Geometry: final body of the model. Coordinates: model frame, mm. A direction names the side the tool comes from. Give positions to 0.01 mm unless a question says otherwise; leave off trailing zeros. Write each loop counter-clockwise with the first axis right and the second up, starting at its lowest first coordinate (ties: lowest second). Pieces come first, ordered by that corner, then holes.
```python
from build123d import *

# Parameters (mm, degrees)
SKETCH1_W           = 96.52
SKETCH1_H           = 72.39
BOSS_EXTRUDE1_DEPTH = 5.08
SHELL1_T            = -2.667
FILLET1_R           = 6.35
FILLET2_R           = 8.89
SKETCH2_W           = 36.83
SKETCH2_H           = 2.413
CUT_EXTRUDE1_DEPTH  = 5.08
SKETCH3_W           = 17.78
SKETCH3_H           = 2.413
CUT_EXTRUDE2_DEPTH  = 5.08
FILLET3_R           = 0.508
CUT_EXTRUDE3_REACH  = 7.08
SKETCH4_R           = 3.25
CUT_EXTRUDE4_DEPTH  = 6.08


with BuildPart() as part:
    # Sketch1 → Boss-Extrude1 (new body)
    with BuildSketch(Plane(origin=(0, 0, 0), x_dir=(1, 0, 0), z_dir=(0, 1, 0))):
        Rectangle(SKETCH1_W, SKETCH1_H)
    extrude(amount=BOSS_EXTRUDE1_DEPTH)

    # Shell1
    shell1_openings = [part.faces().sort_by_distance(p)[0] for p in [
        (0, 5.08, 0),
    ]]
    offset(amount=SHELL1_T, openings=shell1_openings, kind=Kind.INTERSECTION)

    # Fillet1
    fillet1_edges = [part.edges().sort_by_distance(p)[0] for p in [
        (45.593, 3.8735, 33.528),
        (45.593, 3.8735, -33.528),
        (-45.593, 3.8735, -33.528),
        (-45.593, 3.8735, 33.528),
    ]]
    fillet(fillet1_edges, radius=FILLET1_R)

    # Fillet2
    fillet2_edges = [part.edges().sort_by_distance(p)[0] for p in [
        (48.26, 2.54, 36.195),
        (-48.26, 2.54, 36.195),
        (-48.26, 2.54, -36.195),
        (48.26, 2.54, -36.195),
    ]]
    fillet(fillet2_edges, radius=FILLET2_R)

    # Sketch2 → Cut-Extrude1 (cut)
    with BuildSketch(Plane.XY.offset(36.195)):
        with Locations((17.145, 3.8735)):
            Rectangle(SKETCH2_W, SKETCH2_H)
    extrude(amount=-CUT_EXTRUDE1_DEPTH, mode=Mode.SUBTRACT)

    # Sketch3 → Cut-Extrude2 (cut)
    with BuildSketch(Plane(origin=(0, 0, -36.195), x_dir=(-1, 0, 0), z_dir=(0, 0, -1))):
        with Locations((-25.654, 3.8735)):
            Rectangle(SKETCH3_W, SKETCH3_H)
    extrude(amount=-CUT_EXTRUDE2_DEPTH, mode=Mode.SUBTRACT)

    # Fillet3
    fillet3_edges = [part.edges().sort_by_distance(p)[0] for p in [
        (34.544, 2.667, -34.8615),
        (34.544, 5.08, -34.8615),
        (16.764, 5.08, -34.8615),
        (16.764, 2.667, -34.8615),
        (35.56, 5.08, 34.8615),
        (35.56, 2.667, 34.8615),
        (-1.27, 2.667, 34.8615),
        (-1.27, 5.08, 34.8615),
    ]]
    fillet(fillet3_edges, radius=FILLET3_R)

    # Sketch4 → Cut-Extrude3 (cut, up to next)
    with BuildSketch(Plane.XZ, mode=Mode.PRIVATE) as cut_extrude3_sk1:
        with Locations((-38.231636466, 7.223235777)):
            Circle(SKETCH4_R)
    cut_extrude3_tool1 = extrude(cut_extrude3_sk1.sketch, amount=-CUT_EXTRUDE3_REACH, mode=Mode.PRIVATE) & part.part
    add(cut_extrude3_tool1.solids().sort_by_distance((-38.231636, 0, 7.223236))[0], mode=Mode.SUBTRACT)
    # Sketch4 → Cut-Extrude3 (cut, up to next)
    with BuildSketch(Plane.XZ, mode=Mode.PRIVATE) as cut_extrude3_sk2:
        with Locations((12.830494848, -12.70407972)):
            Circle(SKETCH4_R)
    cut_extrude3_tool2 = extrude(cut_extrude3_sk2.sketch, amount=-CUT_EXTRUDE3_REACH, mode=Mode.PRIVATE) & part.part
    add(cut_extrude3_tool2.solids().sort_by_distance((12.830495, 0, -12.70408))[0], mode=Mode.SUBTRACT)

    # Sketch5 → Cut-Extrude4 (cut, through all)
    with BuildSketch(Plane.XZ):
        with BuildLine():
            Line((-9.530108749, 10.470046155), (-9.530108749, -14.929953845))
            ThreePointArc((-9.530108749, -14.929953845), (-12.705108749, -18.104953845), (-15.880108749, -14.929953845))
            Line((-15.880108749, -14.929953845), (-15.880108749, 10.470046155))
            ThreePointArc((-15.880108749, 10.470046155), (-12.705108749, 13.645046155), (-9.530108749, 10.470046155))
        make_face()
        with BuildLine():
            Line((3.169891251, 10.470046155), (3.169891251, -14.929953845))
            ThreePointArc((3.169891251, -14.929953845), (-0.005108749, -18.104953845), (-3.180108749, -14.929953845))
            Line((-3.180108749, -14.929953845), (-3.180108749, 10.470046155))
            ThreePointArc((-3.180108749, 10.470046155), (-0.005108749, 13.645046155), (3.169891251, 10.470046155))
        make_face()
        with BuildLine():
            Line((-22.230108749, 10.470046155), (-22.230108749, -14.929953845))
            ThreePointArc((-22.230108749, -14.929953845), (-25.405108749, -18.104953845), (-28.580108749, -14.929953845))
            Line((-28.580108749, -14.929953845), (-28.580108749, 10.470046155))
            ThreePointArc((-28.580108749, 10.470046155), (-25.405108749, 13.645046155), (-22.230108749, 10.470046155))
        make_face()
    extrude(amount=-CUT_EXTRUDE4_DEPTH, mode=Mode.SUBTRACT)


solid = part.part
```
Item 1: Section B-B, the plane z = -22. Return the cut outline in (x, y).
Found:
outline: (-48.26, 0) - (48.26, 0) - (48.26, 5.08) - (45.59, 5.08) - (45.59, 2.67) - (-45.59, 2.67) - (-45.59, 5.08) - (-48.26, 5.08) - close
Item 2: Section A-A, the plane x = -38. Return the cut outline in (y, z) (1 decimal), plus the area to 3 significant figures.
Found:
outline: (0, -36.2) - (5.1, -36.2) - (5.1, -33.5) - (2.7, -33.5) - (2.7, 4) - (0, 4) - close; (0, 10.5) - (2.7, 10.5) - (2.7, 33.5) - (5.1, 33.5) - (5.1, 36.2) - (0, 36.2) - close
area: 189 mm2
Item 3: Section C-C, the plane y = 1.8. State how many separate pieces and enclosed holes the cut face has, plus the area to 3 significant figures.
Found:
separate pieces: 1
enclosed holes: 5
area: 6,270 mm2
Item 4: Pull-direction query (Z, two-part tool) for faces 4 (the face through (48.26, 3, 0)), 5 (the face through (-43.8, 3.9, -31.6)), 6 (the face through (-3.18, 1, -2)), 7 (the face through (-45.725, 2.576, -33.522)); classes: +Z half, -Z half, draft (parallel to the pull), parting line (faces both ways), or undercut.
Found:
face 4: draft
face 5: undercut
face 6: undercut
face 7: -Z half
Item 5: Pin query (flat end, axial travel): pin 1 Ø1.5 at (y, z) = (3.5, -35) entering from -X; pin 2 Ø2 at (x, z) = (20, 4) entering from +Y; pin 3 Ø6 at (x, z) = (-38.23, 7.22) entering from -Y; pin 4 Ø1.5 at (y, z) = (4, -34) entering from +X. Return the tip coordinate at first contact, or that it passes through.
Found:
pin 1: stops at x = -44.92
pin 2: stops at y = 2.67
pin 3: passes through
pin 4: stops at x = 45.98
Item 6: Reachability of faces 1 (the face through (45.587, 2.576, 33.66)), 2 (the face through (-12.775, 1.315, 13.644)), 3 (the face through (11, 2.667, -1)) from +Z, -Z, +X, -X, +Y, -Y: full face, straight path, thin tool, end or side. Return the list, or none.
Found:
face 1: +Z, +X, +Y, -Y
face 2: +Y, -Y
face 3: +Y
Item 7: Line query: L1, parallel to X at y = 0.9, z = -7; L2, parallel to X at y = 4.2, z = 14; L3, parallel to Z at x = -20.5, y = 4.45 (3 decimals). Output: solid intervals per line, ascending.
Found:
L1: x = -48.26 to -28.58, -22.23 to -15.88, -9.53 to -3.18, 3.17 to 48.26
L2: x = -48.26 to -45.59, 45.59 to 48.26
L3: z = -36.195 to -33.528, 33.528 to 36.195
Item 8: Section D-D, the plane x = 13. Return the cut outline in (y, z) (1 decimal), plus the area to 3 significant figures.
Found:
outline: (0, -36.2) - (5.1, -36.2) - (5.1, -33.5) - (2.7, -33.5) - (2.7, -15.9) - (0, -15.9) - close; (0, -9.5) - (2.7, -9.5) - (2.7, 36.2) - (0, 36.2) - close
area: 182 mm2
